Source: CAD feature listing. Evaluate the final solid. Frame: model axes, mm. A direction names the side the tool comes from. Give positions to 0.01 mm unless a question says otherwise; leave off trailing zeros. Order: outer loops, then holes, each group sorted by start corner. A loop starts at its lowest first (then second) coordinate and runs counter-clockwise, first axis right, second up.
```python
from build123d import *

# Parameters (mm, degrees)
SKETCH1_W                = 107
SKETCH1_H                = 87.7
BOSS_EXTRUDE1_DEPTH      = 13.85
SKETCH2_W                = 102.38
SKETCH2_H                = 83.08
CUT_EXTRUDE1_DEPTH       = 7.9
SKETCH4_R                = 2.5
SKETCH4_R_2              = 1.2
BOSS_EXTRUDE2_DEPTH      = 6.2
SKETCH7_W                = 11.25
SKETCH7_H                = 4.8
BOSS_EXTRUDE3_DEPTH      = 1.7
BOSS_EXTRUDE4_DEPTH      = 3.15
SKETCH9_W                = 12.045425082
SKETCH9_H                = 7.003710523
BOSS_EXTRUDE9_DEPTH      = 5
SKETCH14_W               = 3.501855262
SKETCH14_H               = 2.5
CUT_EXTRUDE6_DEPTH       = 118.146852284
CHAMFER1_SIZE            = 1.5
CHAMFER1_OF_MIRROR4_SIZE = 1.5
MIRROR5_START            = -53.5
MIRROR5_DEPTH            = 12.045425082
BOSS_EXTRUDE10_DEPTH     = 5


# Read off the part's stored shape, not the designer's step: Mirror5
with BuildPart() as part:
    # Sketch1 → Boss-Extrude1 (new body)
    with BuildSketch(Plane(origin=(0, 0, 0), x_dir=(1, 0, 0), z_dir=(0, 1, 0))):
        Rectangle(SKETCH1_W, SKETCH1_H)
    extrude(amount=BOSS_EXTRUDE1_DEPTH)

    # Sketch2 → Cut-Extrude1 (cut)
    with BuildSketch(Plane(origin=(0, 13.85, 0), x_dir=(1, 0, 0), z_dir=(0, 1, 0))):
        Rectangle(SKETCH2_W, SKETCH2_H)
    extrude(amount=-CUT_EXTRUDE1_DEPTH, mode=Mode.SUBTRACT)

    # Sketch4 → Boss-Extrude2 (add)
    # profile 1 of 2: a face of its own
    with BuildSketch(Plane(origin=(0, 5.95, 0), x_dir=(1, 0, 0), z_dir=(0, 1, 0))):
        with Locations(Location((-42.5, -25, 0), (0, 0, 90))):
            Circle(SKETCH4_R)
        with Locations(Location((-42.5, -25, 0), (0, 0, 90))):
            Circle(SKETCH4_R_2, mode=Mode.SUBTRACT)
    # profile 2 of 2: a face of its own
    with BuildSketch(Plane(origin=(0, 5.95, 0), x_dir=(1, 0, 0), z_dir=(0, 1, 0))):
        with Locations(Location((42.5, 25, 0), (0, 0, 90))):
            Circle(SKETCH4_R)
        with Locations(Location((42.5, 25, 0), (0, 0, 90))):
            Circle(SKETCH4_R_2, mode=Mode.SUBTRACT)
    extrude(amount=BOSS_EXTRUDE2_DEPTH)

    # Sketch7 → Boss-Extrude3 (add)
    with BuildSketch(Plane(origin=(-51.19, 0, 0), x_dir=(0, 0, -1), z_dir=(1, 0, 0))):
        with Locations((0, 8.35)):
            Rectangle(SKETCH7_W, SKETCH7_H)
    boss_extrude3 = extrude(amount=BOSS_EXTRUDE3_DEPTH)

    # Sketch8 → Boss-Extrude4 (add, symmetric)
    with BuildSketch(Plane.XY):
        Polygon((-49.49, 10.75), (-49.49, 18.75), (-50.99, 18.75), (-51.99, 16.75), (-51.19, 16.75), (-51.19, 10.75), align=None)
    boss_extrude4 = extrude(amount=BOSS_EXTRUDE4_DEPTH, both=True)

    # Mirror1: Boss-Extrude3, Boss-Extrude4 across plane
    add(boss_extrude3.mirror(Plane(origin=(0, 0, 0), x_dir=(0, 0, 1), z_dir=(1, 0, 0))))
    add(boss_extrude4.mirror(Plane(origin=(0, 0, 0), x_dir=(0, 0, 1), z_dir=(1, 0, 0))))

    # Sketch9 → Boss-Extrude9 (add)
    with BuildSketch(Plane.XZ):
        with Locations((47.477287459, -21.001855262)):
            Rectangle(SKETCH9_W, SKETCH9_H)
    boss_extrude9 = extrude(amount=BOSS_EXTRUDE9_DEPTH)

    # Sketch14 → Cut-Extrude6 (cut, through all)
    with BuildSketch(Plane(origin=(53.5, 0, 0), x_dir=(0, 0, -1), z_dir=(1, 0, 0))):
        with Locations((19.250927631, -1.25)):
            Rectangle(SKETCH14_W, SKETCH14_H)
    cut_extrude6 = extrude(amount=-CUT_EXTRUDE6_DEPTH, mode=Mode.SUBTRACT)

    # Chamfer1
    chamfer1_edges = [part.edges().sort_by_distance(p)[0] for p in [
        (47.477287459, -2.5, -17.5),
    ]]
    chamfer(chamfer1_edges, length=CHAMFER1_SIZE)

    # Mirror4: Boss-Extrude9, Cut-Extrude6 across plane
    add(boss_extrude9.mirror(Plane.XY))
    add(cut_extrude6.mirror(Plane.XY), mode=Mode.SUBTRACT)

    # Chamfer1 of Mirror4
    chamfer1_of_mirror4_edges = [part.edges().sort_by_distance(p)[0] for p in [
        (47.477287459, -2.5, 17.5),
    ]]
    chamfer(chamfer1_of_mirror4_edges, length=CHAMFER1_OF_MIRROR4_SIZE)

    # Mirror5 outline → Mirror5 (add)
    with BuildSketch(Plane.YZ.offset(MIRROR5_START)):
        Polygon((-2.5, -19), (-4, -17.5), (-5, -17.5), (-5, -24.503710523), (0, -24.503710523), (0, -21.001855262), (-2.5, -21.001855262), align=None)
        Polygon((-2.5, 21.001855262), (0, 21.001855262), (0, 24.503710523), (-5, 24.503710523), (-5, 17.5), (-4, 17.5), (-2.5, 19), align=None)
    extrude(amount=MIRROR5_DEPTH)

    # Sketch15 → Boss-Extrude10 (add)
    with BuildSketch(Plane(origin=(0, 0, 0), x_dir=(-1, 0, 0), z_dir=(0, -1, 0))):
        Polygon((-47.477287459, 24.503710523), (-47.477287459, 36.197250384), (48.282556023, 36.197250384), (48.282556023, 24.503710523), (53.5, 24.503710523), (53.5, 43.85), (-53.5, 43.85), (-53.5, 24.503710523), align=None)
    boss_extrude10 = extrude(amount=BOSS_EXTRUDE10_DEPTH)

    # Mirror6: Boss-Extrude10 across plane
    add(boss_extrude10.mirror(Plane.XY))


solid = part.part
```
1) Reachability of faces 5 (the flat face through (47.477, -2, 30)), 6 (the flat face through (-1, 5, -43.85)), 7 (the flat face through (42, 5.95, -25)) from +Z, -Z, +X, -X, +Y, -Y: full face, straight path, thin tool, end or side. Return the list, or none.
Report:
face 5: -Y
face 6: -Z, +X, -X, +Y, -Y
face 7: +Y
2) Material intervals for L1, parallel to Z at x = -42.5, y = 10.5; L2, parallel to Z at x = 42.5, y = 9; L3, parallel to Z at x = -26.5, y = -2.25, sorted ascending.
Report:
L1: z = -43.85 to -41.54, 22.5 to 23.8, 26.2 to 27.5, 41.54 to 43.85
L2: z = -43.85 to -41.54, -27.5 to -26.2, -23.8 to -22.5, 41.54 to 43.85
L3: z = -43.85 to -36.2, 36.2 to 43.85
3) Section query B-B, the plane x = 30. Return the cut outline in (y, z), and give its area (3 significant figures).
Report:
outline: (-5, -43.85) - (13.85, -43.85) - (13.85, -41.54) - (5.95, -41.54) - (5.95, 41.54) - (13.85, 41.54) - (13.85, 43.85) - (-5, 43.85) - (-5, 36.2) - (0, 36.2) - (0, -36.2) - (-5, -36.2) - close
area: 635 mm2
4) Draft query along Y for faces 1 (the flat face through (-41, 12.15, 26)), 2 (the flat face through (48, -1, 21.002)), 3 (the flat face through (41.455, -3, 22)), 4 (the flat face through (51.19, 15, 0)). Return one class per face: +Y half, -Y half, draft (parallel to the pull), parting line (faces both ways), or undercut.
Report:
face 1: +Y half
face 2: undercut
face 3: draft
face 4: undercut
5) Pin query (flat end, axial travel): pin 1 (1.6 mm diameter, centred on x = -46.5, z = 20, fed in from +Y); pin 2 (2 mm diameter, centred on x = 14.5, z = 22.5, fed in from +Y); pin 3 (1.5 mm diameter, centred on y = 15, z = 2.5, fed in from +X). Return the tip coordinate at first contact, or that it passes through.
Report:
pin 1: stops at y = 5.95
pin 2: stops at y = 5.95
pin 3: stops at x = 51.19
6) Section query A-A, the plane y = 15.25. Return the cut outline in (x, z), and give its area (3 significant figures).
Report:
outline: (-51.19, -3.15) - (-49.49, -3.15) - (-49.49, 3.15) - (-51.19, 3.15) - close; (49.49, -3.15) - (51.19, -3.15) - (51.19, 3.15) - (49.49, 3.15) - close
area: 21.4 mm2
7) Section query C-C, the plane z = -1. Return the cut outline in (x, y), and give its area (3 significant figures).
Report:
outline: (-53.5, 0) - (53.5, 0) - (53.5, 13.85) - (51.19, 13.85) - (51.19, 16.75) - (51.99, 16.75) - (50.99, 18.75) - (49.49, 18.75) - (49.49, 5.95) - (-49.49, 5.95) - (-49.49, 18.75) - (-50.99, 18.75) - (-51.99, 16.75) - (-51.19, 16.75) - (-51.19, 13.85) - (-53.5, 13.85) - close
area: 718 mm2
